Read the model definition and answer for the solid it produces. Units are mm, in the model's axes. A direction names the side the tool comes from. Coordinates: 2 decimals unless noted, no trailing zeros. Write each loop counter-clockwise with the first axis right and the second up, starting at its lowest first coordinate (ties: lowest second). Pieces come first, ordered by that corner, then holes.
Item 1: Section C-C (z = -41) is taken. Give the vertices of the cut face in (x, y) (3 decimals), then the cut area to 3 significant figures.
Item 2: Section A-A (y = 0) is taken. Give the vertices of the cut face in (x, z), then the cut area to 3 significant figures.
Item 3: Straight lines are drawn through the part: probe 1 along Z at (x, y) = (-87.5, -151); probe 2 along Y at (x, z) = (-80, -116); probe 3 along Z at (x, y) = (127, -28). For each, find the intervals that lie inside material, in ascending order.
Item 4: Section D-D (z = 89) is taken. Give the vertices of the cut face in (x, y), then the cut area to 3 significant figures.
Item 5: Determine the mould class of faces 1 (the face through (-81.63, -126.17, 117.6)), 2 (the face through (-94.425, -164.868, -117.605)), 3 (the face through (52.388, 144.461, 8.459)), 4 (the face through (79.749, 161.803, 26.062)) for opening direction X: released by +X, released by -X, zero draft, split by the parting line, or undercut.
Item 6: Section B-B (x = -80) is taken. Give the vertices of the cut face in (y, z), then the cut area to 3 significant figures.
Item 7: Each of these flat-tipped pins is pushed along its axis until it touches: P1, Ø10, axis at y = 83.5, z = 73, coming from the -X side; P2, Ø12, axis at x = 144, z = 116.5, coming from the -Y side; P3, Ø12, axis at x = 52.5, z = 74, coming from the +Y side. Where does it stop, or does it pass through?
Item 8: A tool of negligible diameter and unlimited length cuts with its end or side. For faces 5 (the face through (20.435, -147.077, -23.153)), 6 (the face through (83, -58, 125)), 7 (the face through (140, -30, 118)), 8 (the face through (-65, 130, 110)), 9 (the face through (-96.17, -106.57, 117.6)), from which of +Z, -Z, +X, -X, +Y, -Y can it reach the whole face along a straight path? Write none if from no direction.
from build123d import *

# Parameters (mm, degrees)
F1_R             = 125
F1_R_2           = 100
F2_DEPTH         = 250
F3_R             = 12.5
F4_DEPTH         = 15
F4_COPIES_COUNT  = 3
F4_COPIES1_COUNT = 2
F10_R            = 56.8493867215
F10_R_2          = 5
F10_R_3          = 28.1619206838
F11_DEPTH        = 68.6754869442
F15_R            = 60.4503373428
F18_D            = 8.5
F18_CBORE_D      = 17.25
F18_CBORE_DEPTH  = 10


# Not quite as in the source:
# - ends of sketch curves that miss each other by under 0.0002 mm in the source are joined
# - a pattern or mirror of a feature is missing from the dataset's text; its kind, count and spacing are read off the source's solid


with BuildPart() as f2:
    # F1 (on offset) → F2 (new body)
    with BuildSketch(Plane.XY.offset(125)):
        Circle(F1_R)
        Circle(F1_R_2, mode=Mode.SUBTRACT)
    extrude(amount=-F2_DEPTH)

    # F3 (on face) → F4 (join)
    with BuildSketch(Plane.XY.offset(125)):
        with BuildLine():
            Line((-105.9807621135, 123.5640646055), (-86.6540676111, 90.0892477849))
            ThreePointArc((-86.6540676111, 90.0892477849), (-62.5, 108.2531754731), (-34.692543384, 120.0892477849))
            Line((-34.692543384, 120.0892477849), (-53.9970505647, 153.5256350369))
            ThreePointArc((-53.9970505647, 153.5256350369), (-54.008151328, 153.5448457136), (-54.0192378865, 153.5640646055))
            ThreePointArc((-54.0192378865, 153.5640646055), (-95, 164.544826719), (-105.9807621135, 123.5640646055))
        make_face()
        with Locations((-80, 138.5640646055)):
            Circle(F3_R, mode=Mode.SUBTRACT)
    f4 = extrude(amount=-F4_DEPTH)

    # F4_copies: F4 ×3 about axis
    f4_copies_axis = Axis((0, 0, 0), (0, 0, 1))
    for i in range(1, F4_COPIES_COUNT):
        add(f4.rotate(f4_copies_axis, i * 360 / F4_COPIES_COUNT))

    # F4_copies1: F4 ×2 about axis
    f4_copies1_axis = Axis((0, 0, 0), (1, 0, 0))
    for i in range(1, F4_COPIES1_COUNT):
        add(f4.rotate(f4_copies1_axis, i * 360 / F4_COPIES1_COUNT))

    # F10 (on offset) → F11 (join, through all)
    with BuildSketch(Plane(origin=(90, 155.8845726812, 0), x_dir=(-0.8660254038, 0.5, 0), z_dir=(0.5, 0.8660254038, 0))):
        Circle(F10_R)
        with Locations((-36.7784088222, -21.2340242338)):
            Circle(F10_R_2, mode=Mode.SUBTRACT)
        with Locations((36.7784088222, -21.2340242338)):
            Circle(F10_R_2, mode=Mode.SUBTRACT)
        Circle(F10_R_3, mode=Mode.SUBTRACT)
        with Locations((0, 42.4680484677)):
            Circle(F10_R_2, mode=Mode.SUBTRACT)
    extrude(amount=-F11_DEPTH)

    # F15 (on offset) → F16 (join, up to the next surface of F2)
    with BuildSketch(Plane(origin=(77.4998450043, -134.2344088806, 0), x_dir=(-0.8660265969, -0.4999979334, 0), z_dir=(-0.4999979334, 0.8660265969, 0))):
        Circle(F15_R)
    extrude(until=Until.NEXT)

    # F18 (through all)
    with Locations(Plane(origin=(77.4998450043, -134.2344088806, 0), x_dir=(0.8660265969, 0.4999979334, 0), z_dir=(0.4999979334, -0.8660265969, 0))):
        with Locations((0, 0)):
            CounterBoreHole(F18_D / 2, F18_CBORE_D / 2, F18_CBORE_DEPTH)


solid = f2.part
Established:
1. outline: (19.95, -123.398) - (39.03, -156.445) - (115.97, -112.024) - (96.89, -78.977) arc R125 ccw to (93.422, 83.05) - (124.105, 136.194) - (55.895, 175.575) - (25.212, 122.431) arc R125 ccw (long way) to start; hole circle Ø200 at (0, 0)
1. area: 25,100 mm2
2. outline: (-125, -125) - (-100, -125) - (-100, 125) - (-125, 125) - close; (100, -125) - (125, -125) - (125, 110) - (147.5, 110) - (147.5, 125) - (100, 125) - close; (172.5, 110) - (190, 110) - (190, 125) - (172.5, 125) - close
2. area: 13,100 mm2
3. probe 1: z = -125 to -110, 110 to 125
3. probe 2: y = -168.56 to -151.06, -126.06 to -60, 60 to 96.05
3. probe 3: z = 110 to 125
4. outline: circle Ø250 at (0, 0); hole circle Ø200 at (0, 0)
4. area: 17,700 mm2
5. face 1: undercut
5. face 2: split by the parting line
5. face 3: undercut
5. face 4: released by +X
6. outline: (-168.56, -125) - (-151.06, -125) - (-151.06, -110) - (-168.56, -110) - close; (-168.56, 110) - (-151.06, 110) - (-151.06, 125) - (-168.56, 125) - close; (-126.06, -125) - (-60, -125) - (-60, 125) - (-126.06, 125) - (-126.06, 110) - (-96.05, 110) - (-96.05, -110) - (-126.06, -110) - close; (60, -125) - (96.05, -125) - (96.05, 110) - (126.06, 110) - (126.06, 125) - (60, 125) - close; (151.06, 110) - (168.56, 110) - (168.56, 125) - (151.06, 125) - close
6. area: 20,200 mm2
7. P1: stops at x = -97.28
7. P2: stops at y = -30
7. P3: stops at y = 116.03
8. face 5: none
8. face 6: +Z, +X, -X, +Y, -Y
8. face 7: +Z, -Z, +X, -Y
8. face 8: -Z, -X, +Y
8. face 9: +Z, -Z, -X
